Drawing for the job (mm, zero at the part's lowest x, y, z). Coordinates: 2 decimals unless noted, no trailing zeros. Write each loop counter-clockwise with the first axis right and the second up, starting at its lowest first coordinate (ties: lowest second). Pieces come first, ordered by that corner, then holes. Notation, with made-up numbers: (10.25, 58.25) -> (56.25, 58.25) arc R20 ccw to (56.25, 89.25) -> close; hole circle Ø4 at (45, 78). An arc over 180 degrees is marked (long way). Answer as CSV lines item,"result". Start each with the question number.
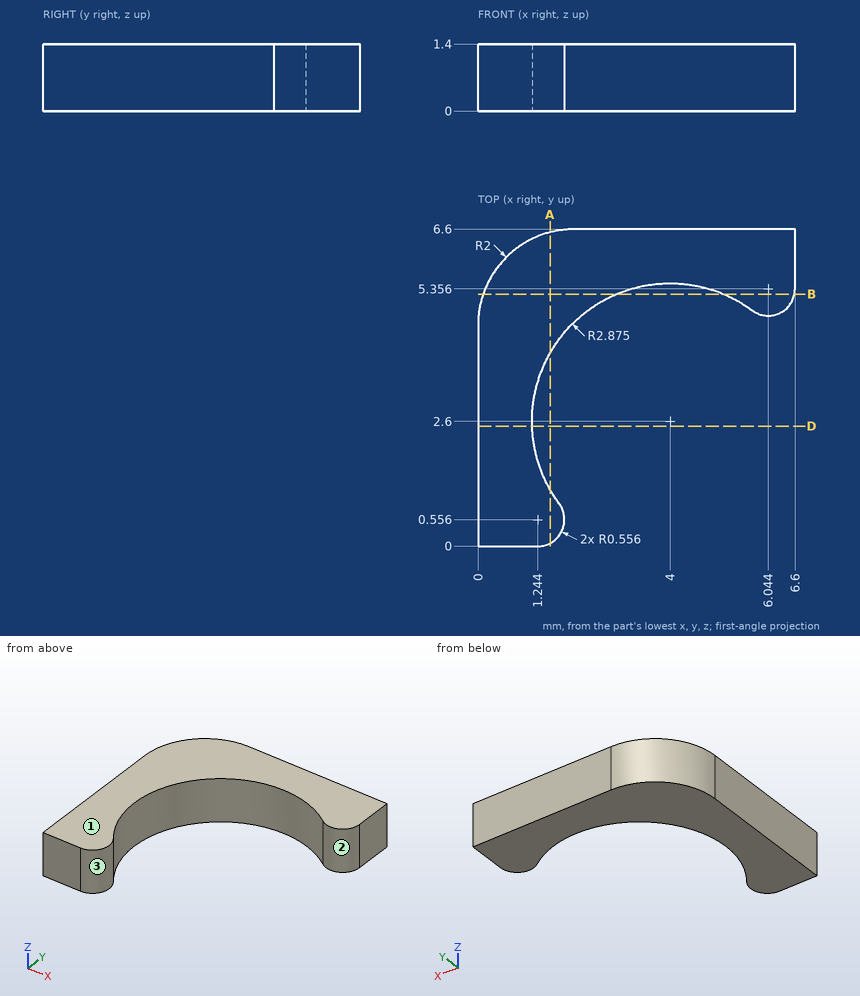
1. Wall check: line 1 (Y direction, x = 1.5, z = 0.1) (1 decimal); line 2 (Y direction, x = 6, z = 0.95); line 3 (X direction, y = 0.5, z = 0.2). Give the ranges that are in metal, low to high.
2. Cut at D-D (y = 2.5). Give the cut face in (x, z).
3. Mould opens along X. For the marked faces 1, 2 and 3 say: pulls with the +X half, pulls with the -X half, needs draft (parallel to the pull), parting line crosses it, or undercut.
4. Cut at A-A (x = 1.5). Give the cut face in (y, z).
5. Cut at B-B (y = 5.25). Give the cut face in (x, z) (1 decimal).
Geometry check:
1,line 1,"0.1 to 1.2, 4 to 6.5"
1,line 2,"4.8 to 6.6"
1,line 3,"0 to 1.8"
2,outline,"(0, 0) -> (1.13, 0) -> (1.13, 1.4) -> (0, 1.4) -> close"
3,face 1,"needs draft"
3,face 2,"undercut"
3,face 3,"pulls with the +X half"
4,outline,"(0.06, 0) -> (1.18, 0) -> (1.18, 1.4) -> (0.06, 1.4) -> close; (4.02, 0) -> (6.54, 0) -> (6.54, 1.4) -> (4.02, 1.4) -> close"
5,outline,"(0.1, 0) -> (2.9, 0) -> (2.9, 1.4) -> (0.1, 1.4) -> close; (5.1, 0) -> (6.6, 0) -> (6.6, 1.4) -> (5.1, 1.4) -> close"
